CAD build for the part. Positions are in the model's coordinates, mm. Give positions to 0.01 mm unless a question says otherwise; leave off trailing zeros. Write each loop counter-clockwise with the first axis right and the second up, starting at its lowest first coordinate (ties: lowest second). Pieces come first, ordered by that corner, then holes. Notation, with made-up numbers: (-21, 29.5) - (13, 29.5) arc R14 cw to (13, 44.5) - close; hole circle Ø9 at (63, 51). An arc over 180 degrees is marked (long way). Answer as a JSON object with one key per item and string values.
from build123d import *

# Parameters (mm, degrees)
F0_R     = 25
F1_DEPTH = 3
F2_R     = 2


# Not quite as in the source:
# - a fillet or chamfer that OpenCascade refuses, or shapes differently, is made with other operations: its cross-section is extruded or revolved along the edge and cut away or added


with BuildPart() as f1:
    # F0 (on Top) → F1 (new body, symmetric)
    with BuildSketch(Plane.XY):
        Circle(F0_R)
    extrude(amount=F1_DEPTH, both=True)

    # F2
    f2_edges = [f1.edges().sort_by_distance(p)[0] for p in [
        (-25, 0, 3),
    ]]
    fillet(f2_edges, radius=F2_R)

    # F3: chamfer of 5 on 1 edges, made by hand

    # F3_s1 → F3_t2 (revolve, cut)
    with BuildSketch(Plane.XZ):
        Polygon((25, 2), (20, -3), (25, -3), align=None)
    revolve(axis=Axis((0, 0, -3), (0, 0, 1)), mode=Mode.SUBTRACT)


solid = f1.part
Item 1: Cut at A-A (y = 0). Give the cut face in (x, z).
Entries:
{"outline": "(-24.82, 1.82) - (-20, -3) - (20, -3) - (24.82, 1.82) arc R2 ccw to (23, 3) - (-23, 3) arc R2 ccw to start"}
Item 2: Flat gauge pins, fed straight in: P1, Ø1.5, axis at y = 1.5, z = 1.5, coming from the -X side; P2, Ø3, axis at y = -17, z = 1.5, coming from the -X side; P3, Ø1, axis at x = 0, z = -1.5, coming from the -Y side. Where does each tip first touch, or does it go through?
Entries:
{"P1": "x = -24.81", "P2": "x = -19.36", "P3": "y = -22"}
Item 3: Probe line 1 (X direction, y = -20.5, z = 1.5); line 2 (Y direction, x = -7, z = 1.25); line 3 (Y direction, x = 16, z = -1). List the from-to ranges inside material, lowest first. Write a range as from..to.
Entries:
{"line 1": "-13.42..13.42", "line 2": "-23.22..23.22", "line 3": "-15.1..15.1"}
Item 4: Cut at D-D (z = -2.25). Give the cut face in (x, y).
Entries:
{"outline": "circle Ø41.5 at (0, 0)"}
Item 5: Cut at C-C (z = 0.5). Give the cut face in (x, y).
Entries:
{"outline": "circle Ø47 at (0, 0)"}
